```python
from build123d import *

# Parameters (mm, degrees)
SKETCH1_R           = 10
BOSS_EXTRUDE1_DEPTH = 10
FILLET1_R           = 3


with BuildPart() as part:
    # Sketch1 → Boss-Extrude1 (new, symmetric)
    with BuildSketch(Plane.XY):
        with BuildLine():
            Line((-7.5, 16.459503782), (-7.5, -16.459503782))
            ThreePointArc((-7.5, -16.459503782), (0, -55), (7.5, -16.459503782))
            Line((7.5, -16.459503782), (7.5, 16.459503782))
            ThreePointArc((7.5, 16.459503782), (0, 55), (-7.5, 16.459503782))
        make_face()
        with Locations((0, 35)):
            Circle(SKETCH1_R, mode=Mode.SUBTRACT)
        with Locations(Location((0, -35, 0), (0, 0, 180))):
            Circle(SKETCH1_R, mode=Mode.SUBTRACT)
    extrude(amount=BOSS_EXTRUDE1_DEPTH, both=True)

    # Fillet1
    fillet1_edges = [part.edges().sort_by_distance(p)[0] for p in [
        (0, -55, 10),
        (7.5, 0, 10),
        (0, 55, 10),
        (7.5, 0, -10),
        (0, -55, -10),
        (-7.5, 0, -10),
        (0, 55, -10),
        (7.5, 16.459503782, 0),
        (7.5, -16.459503782, 0),
        (-7.5, -16.459503782, 0),
        (-7.5, 16.459503782, 0),
        (-7.5, 0, 10),
    ]]
    fillet(fillet1_edges, radius=FILLET1_R)


solid = part.part
```
Geometry check sheet. Reference: the model listing, model coordinates, mm. A direction names the side the tool comes from. Give positions to 0.01 mm unless a question says otherwise; leave off trailing zeros. Write each loop counter-clockwise with the first axis right and the second up, starting at its lowest first coordinate (ties: lowest second). Pieces come first, ordered by that corner, then holes. Notation, with made-up numbers: (19, 5.25) -> (33, 5.25) arc R27 ccw to (33, 31.25) -> close; hole circle Ø11 at (19.25, 21). An arc over 180 degrees is marked (long way). Use one line per item in the form item = value.
Item 1: Mould release check, pull along Y, two halves, no side actions. Record for faces 1 (the cylindrical face through (-6.64, -0.2, 9.1)), 2 (the flat face through (0, 1, -10)), 3 (the cylindrical face through (-7.928, -16.081, 0.098)): released by +Y, released by -Y, zero draft, split by the parting line, or undercut.
Results list:
face_1 = undercut
face_2 = zero draft
face_3 = undercut
Item 2: Depth check by flat-ended pin: pin 1 Ø3 at (x, z) = (-2, 6.5) entering from -Y; pin 2 Ø11 at (y, z) = (3.5, -2.5) entering from +X; pin 3 Ø7 at (y, z) = (-1, 3) entering from -X. Enter the tip coordinate at first touch or a pass-through.
Results list:
pin_1 = -54.99
pin_2 = 7.5
pin_3 = -7.5
Item 3: Sectioned sample at C-C on y = 3. Enter the section's corners in (x, z).
Results list:
outline = (-7.5, -7) arc R3 ccw to (-4.5, -10) -> (4.5, -10) arc R3 ccw to (7.5, -7) -> (7.5, 7) arc R3 ccw to (4.5, 10) -> (-4.5, 10) arc R3 ccw to (-7.5, 7) -> close
Item 4: Scan lines: line 1 (X direction, y = -35, z = 2.5); line 2 (Y direction, x = -9, z = -6.25); line 3 (X direction, y = -44, z = 4.75). Record each from-to range of solid material in increasing order.
Results list:
line_1 = -20 to -10, 10 to 20
line_2 = -52.86 to -39.36, -30.64 to -17.13, 17.13 to 30.64, 39.36 to 52.86
line_3 = -17.86 to -4.36, 4.36 to 17.86
Item 5: Access from +Z, -Z, +X, -X, +Y, -Y to the whole of each face (thin tool, end or side, straight path). Record for faces 4 (the flat face through (-7.5, 0, 0)), 5 (the cylindrical face through (6.64, 0.2, 9.1)), 6 (the cylindrical face through (7.95, 16.12, -0.1)), 7 (the cylindrical face through (6.64, 0.2, -9.1)).
Results list:
face_4 = +Z, -Z, -X
face_5 = +Z, +X
face_6 = +Z, -Z, +X
face_7 = -Z, +X
Item 6: Sectioned sample at B-B on z = -5.5. Enter the section's corners in (x, y).
Results list:
outline = (-9.13, -17.21) arc R20 ccw (long way) to (9.13, -17.21) arc R3 cw to (7.5, -14.54) -> (7.5, 14.54) arc R3 cw to (9.13, 17.21) arc R20 ccw (long way) to (-9.13, 17.21) arc R3 cw to (-7.5, 14.54) -> (-7.5, -14.54) arc R3 cw to start; hole circle Ø20 at (0, -35); hole circle Ø20 at (0, 35)
Item 7: Sectioned sample at A-A on x = 0. Enter the section's corners in (y, z).
Results list:
outline = (-55, -7) arc R3 ccw to (-52, -10) -> (-45, -10) -> (-45, 10) -> (-52, 10) arc R3 ccw to (-55, 7) -> close; (-25, -10) -> (25, -10) -> (25, 10) -> (-25, 10) -> close; (45, -10) -> (52, -10) arc R3 ccw to (55, -7) -> (55, 7) arc R3 ccw to (52, 10) -> (45, 10) -> close
